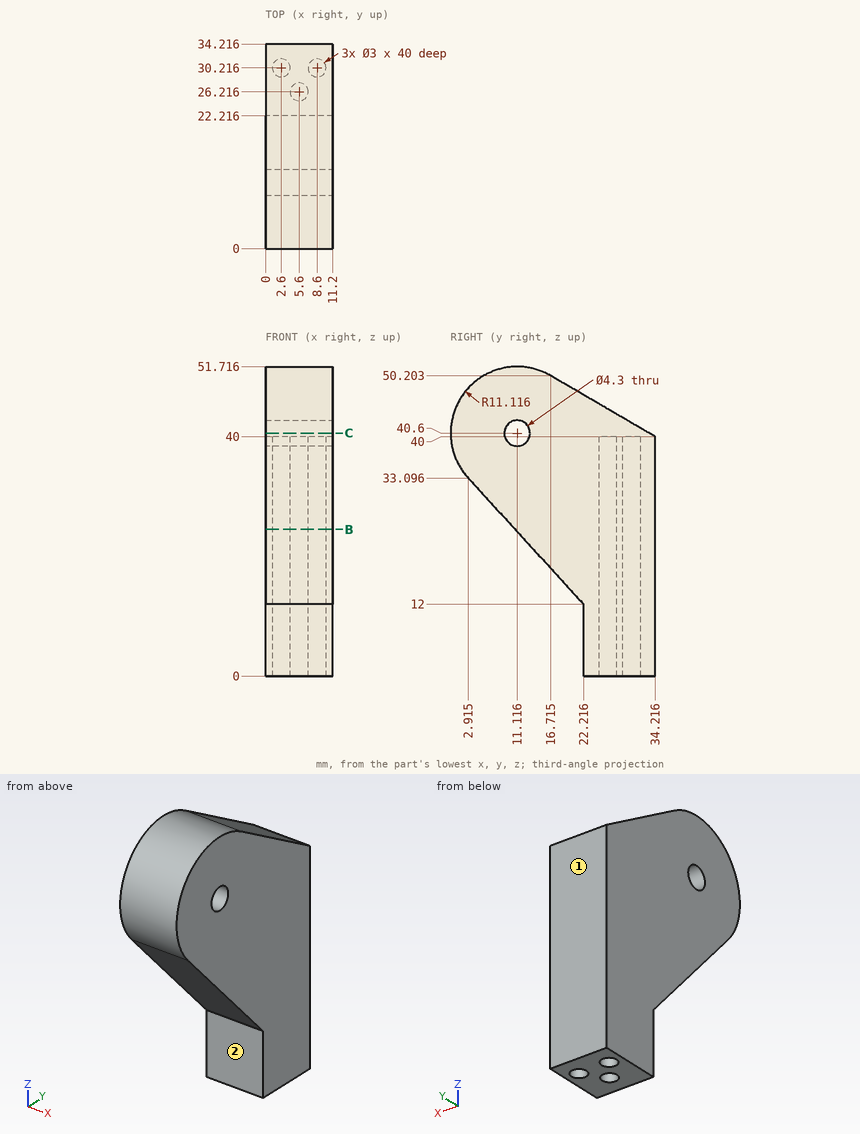
For this review, use the dimensioned drawing (mm, ordinates from the lowest corner) and the shaded views. A direction names the side the tool comes from. Give positions to 0.01 mm unless a question says otherwise; leave off trailing zeros. Loops run counter-clockwise (first coordinate to the right, second up) from the corner with the lowest first, then second, coordinate; pieces in that order, holes last.
Item 1: Insertion check: pin 1 (2 mm diameter, centred on x = 5, y = 24.5, fed in from -Z); pin 2 (2.5 mm diameter, centred on x = 8.6, y = 30.22, fed in from -Z); pin 3 (1 mm diameter, centred on x = 7.5, z = 32, fed in from -Y); pin 4 (2.5 mm diameter, centred on x = 5.6, y = 26.22, fed in from +Z). Each pin has a flat end and moves straight along its axis. Give the tip position at first contact, or say it passes through.
Item 2: For line 1 along Y through (x, z) = (8.6, 18) (1 decimal); line 2 along X through (y, z) = (30.5, 2.5); line 3 along Y through (x, z) = (4.5, 39.5) (1 decimal), list the stretches that pass through material, from the lowest coordinate up.
Item 3: Take a section at C-C, the plane z = 40.6. State the section outline as (x, y) points.
Item 4: Tool access review of the marked faces 1 and 2: name each direction out of +Z, -Z, +X, -X, +Y, -Y from which nothing blocks a thin tool from reaching the whole face with its end or side.
Item 5: Take a section at B-B, the plane z = 24.5. State the section outline as (x, y) points.
Calculated:
1. pin 1: stops at z = 0
1. pin 2: stops at z = 40
1. pin 3: stops at y = 3.46
1. pin 4: stops at z = 45.39
2. line 1: y = 16.7 to 28.7, 31.7 to 34.2
2. line 2: x = 0 to 1.13, 4.07 to 7.13, 10.07 to 11.2
2. line 3: y = 0.1 to 9.3, 13 to 25.2, 27.2 to 34.2
3. outline: (0, 0) - (11.2, 0) - (11.2, 8.97) - (0, 8.97) - close; (0, 13.27) - (11.2, 13.27) - (11.2, 33.19) - (0, 33.19) - close
4. face 1: +Z, -Z, +X, -X, +Y
4. face 2: -Z, +X, -X, -Y
5. outline: (0, 10.78) - (11.2, 10.78) - (11.2, 34.22) - (0, 34.22) - close; hole circle Ø3 at (2.6, 30.22); hole circle Ø3 at (5.6, 26.22); hole circle Ø3 at (8.6, 30.22)
